```python
from build123d import *

# Parameters (mm, degrees)
F1_DEPTH  = 2.95
F2_W      = 2.95
F2_H      = 50
F3_DEPTH  = 2.95
F4_W      = 20
F4_H      = 2.95
F5_DEPTH  = 1.25
F7_D      = 6
F7_DEPTH  = 4
F7_TIP    = 1.8025818571
F8_W      = 30
F8_H      = 1.25
F9_DEPTH  = 2.95
F10_W     = 2.95
F10_H     = 50
F11_DEPTH = 2.95


# Not quite as in the source:
# - a feature names something its author has since deleted; it is built from what else it names


with BuildPart() as f1:
    # F0 (on Front) → F1 (new body)
    with BuildSketch(Plane.XZ):
        Polygon((50, -6), (50, 0), (150, 0), (150, -6), (200, -6), (200, 0), (300, 0), (300, -6), (350, -6), (350, 0), (350, 200), (0, 200), (-50, 200), (-50, 0), (0, 0), (0, -6), align=None)
    extrude(amount=F1_DEPTH)

    # F2 (on face) → F3 (cut)
    with BuildSketch(Plane.XZ.offset(2.95)):
        with Locations((325.4, 150)):
            Rectangle(F2_W, F2_H)
        with Locations((325.4, 67)):
            Rectangle(F2_W, F2_H)
    extrude(amount=-F3_DEPTH, mode=Mode.SUBTRACT)

    # F4 (on face) → F5 (join)
    with BuildSketch(Plane.XY.offset(200)):
        with Locations((80, -1.475)):
            Rectangle(F4_W, F4_H)
        with Locations((30, -1.475)):
            Rectangle(F4_W, F4_H)
        with Locations((-20, -1.475)):
            Rectangle(F4_W, F4_H)
    extrude(amount=F5_DEPTH)

    # F7
    with Locations(Plane(origin=(0, 0, 0), x_dir=(-1, 0, 0), z_dir=(0, 1, 0))):
        with Locations((-80, 91.25), (-80, 191.25), (-30, 91.25), (20, 91.25), (20, 191.25), (-30, 191.25)):
            Hole(F7_D / 2, depth=F7_DEPTH)
            with Locations((0, 0, -(F7_DEPTH + F7_TIP / 2))):  # 118° drill point
                Cone(0, F7_D / 2, F7_TIP, mode=Mode.SUBTRACT)

    # F8 (on face) → F9 (join)
    with BuildSketch(Plane(origin=(0, 0, 0), x_dir=(-1, 0, 0), z_dir=(0, 1, 0))):
        with Locations((-55, 200.625)):
            Rectangle(F8_W, F8_H)
        Polygon((30, 201.25), (30, 200), (50, 200), align=None)
        Polygon((-90, 200), (-90, 201.25), (-110, 200), align=None)
        Polygon((10, 201.25), (-5, 200), (10, 200), align=None)
        Polygon((-8.75, 200), (-20, 201.25), (-20, 200), align=None)
    extrude(amount=-F9_DEPTH)

    # F10 (on face) → F11 (cut)
    with BuildSketch(Plane(origin=(0, 0, 0), x_dir=(-1, 0, 0), z_dir=(0, 1, 0))):
        with Locations((-6.475, 150)):
            Rectangle(F10_W, F10_H)
        with Locations((-6.475, 67)):
            Rectangle(F10_W, F10_H)
    extrude(amount=-F11_DEPTH, mode=Mode.SUBTRACT)


solid = f1.part
```
Could you check a few things on this model? Use its own coordinates, in mm. Round coordinates to 2 decimals unless told otherwise and drop trailing zeros. Loops run counter-clockwise (first coordinate to the right, second up) from the corner with the lowest first, then second, coordinate; pieces in that order, holes last. Notation, with made-up numbers: M -15,51 L 0,51 A23 cw 0,66 Z; hole C -0.75,18.5 d2. An arc over 180 degrees is marked long. Answer as CSV lines item,"result".
1) For pin 1 Ø1 at (x, y) = (116, -1) entering from -Z, with a flat end and sliding along its axis, tell me the tip position at first contact or that it passes through.
From the geometry:
pin 1,"z = 0"
2) Imagine slicing it at A-A on y = -1.25. Count the separate pieces of the cut face and the enclosed holes in it, and give its area (3 significant figures).
From the geometry:
separate pieces,"1"
enclosed holes,"10"
area,"80,300 mm^2"
3) If I drill on probe 1 along Z at (x, y) = (7, -2.8); probe 2 along Z at (x, y) = (30, -1.1); probe 3 along X at (y, z) = (-0.8, 87) (3 decimals), over which ranges is the centre line in solid material (lowest first)?
From the geometry:
probe 1,"-6 to 42, 92 to 125, 175 to 200"
probe 2,"-6 to 88.25, 94.25 to 188.25, 194.25 to 201.25"
probe 3,"-50 to 5, 7.95 to 323.925, 326.875 to 350"
4) Imagine slicing it at B-B on x = 273.5. List the corners of the cut face in (y, z) for me, and give its area (3 significant figures).
From the geometry:
outline,"M -2.95,0 L 0,0 L 0,200 L -2.95,200 Z"
area,"590 mm^2"
